Can you work these out from the model? Positions are in its coordinate system, mm. Face numbers are marked on the shaded views. A direction names the side the tool comes from. Round coordinates to 2 decimals unless told otherwise and drop trailing zeros. Loops run counter-clockwise (first coordinate to the right, second up) from the corner with the lowest first, then second, coordinate; pieces in that order, holes last. Notation, with made-up numbers: M -2,4 L 20,4 A25 ccw 20,38 Z; hole C 28,16 d7. An arc over 180 degrees is marked long. Return JSON: item names as keys, results as strings.
```python
from build123d import *

# Parameters (mm, degrees)
ESQUISSE1_R             = 3
EXTRUSION1_DEPTH        = 39
ESQUISSE2_R             = 1.5
ENL_V_MAT_EXTRU_1_DEPTH = 10


with BuildPart() as part:
    # Esquisse1 → Extrusion1 (new, symmetric)
    with BuildSketch(Plane.XY):
        Circle(ESQUISSE1_R)
    extrude(amount=EXTRUSION1_DEPTH, both=True)

    # Esquisse2 → Enlèv. mat.-Extru.1 (cut)
    with BuildSketch(Plane.XY.offset(39)):
        Circle(ESQUISSE2_R)
    enl_v_mat_extru_1 = extrude(amount=-ENL_V_MAT_EXTRU_1_DEPTH, mode=Mode.SUBTRACT)

    # Symétrie1: Enlèv. mat.-Extru.1 across plane
    add(enl_v_mat_extru_1.mirror(Plane.XY), mode=Mode.SUBTRACT)

    # Esquisse3 → Révolution1 (revolve)
    with BuildSketch(Plane(origin=(0, 0, 0), x_dir=(1, 0, 0), z_dir=(0, 1, 0))):
        with BuildLine():
            Line((0, 3.5), (0, -3.5))
            ThreePointArc((0, -3.5), (3.5, 0), (0, 3.5))
        make_face()
    revolve(axis=Axis((0, 0, -41.019136627), (0, 0, 1)))


solid = part.part
```
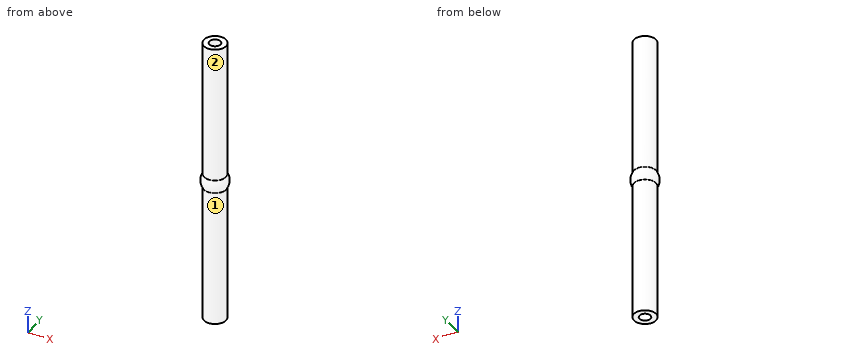
Q1. Suppose I cut it at A-A, the plane z = -31. Please give me the cut outline in (x, y), plus the area to 3 significant figures.
Results:
{"outline": "C 0,0 d6; hole C 0,0 d3", "area": "21.2 mm2"}
Q2. Suppose I cut it at D-D, the plane z = -18. Please give me the cut outline in (x, y), plus the area to 3 significant figures.
Results:
{"outline": "C 0,0 d6", "area": "28.3 mm2"}
Q3. On a 3-axis mill with a long thin cutter (end or side, diameter ignored), from which of +Z, -Z, +X, -X, +Y, -Y can I reach the whole of each face in a straight line? I mean the marked faces 1 and 2. Say none if no direction works.
Results:
{"face 1": "-Z", "face 2": "+Z"}
Q4. I'm going to push flat-ended pins straight in: pin 1 Ø2 at (x, z) = (-1.5, -14) entering from -Y; pin 2 Ø2.5 at (x, y) = (0, 0) entering from -Z; pin 3 Ø3 at (x, z) = (2.5, -19.5) entering from -Y; pin 4 Ø2.5 at (x, y) = (-0.5, 0) entering from -Z. Where does each tip first touch, or does it pass through?
Results:
{"pin 1": "stops at y = -2.96", "pin 2": "stops at z = -29", "pin 3": "stops at y = -2.83", "pin 4": "stops at z = -39"}
Q5. Suppose I cut it at B-B, the plane x = 0. Please give me the cut outline in (y, z), plus the area to 3 significant figures.
Results:
{"outline": "M -3,-39 L -1.5,-39 L -1.5,-29 L 1.5,-29 L 1.5,-39 L 3,-39 L 3,-1.8 A3.5 ccw 3,1.8 L 3,39 L 1.5,39 L 1.5,29 L -1.5,29 L -1.5,39 L -3,39 L -3,1.8 A3.5 ccw -3,-1.8 Z", "area": "410 mm2"}
Q6. If I drill on line 1 along Y through (x, z) = (0, 33.75); line 2 along Z through (x, y) = (0, -1); line 3 along Y through (x, z) = (0, -6), over which ranges is the centre line in solid material (lowest first)?
Results:
{"line 1": "y = -3 to -1.5, 1.5 to 3", "line 2": "z = -29 to 29", "line 3": "y = -3 to 3"}
